```python
from build123d import *

# Parameters (mm, degrees)
SKETCH1_R           = 5
BOSS_EXTRUDE1_DEPTH = 40
CUT_EXTRUDE1_REACH  = 50.283
SKETCH3_W           = 23
SKETCH3_H           = 33
BOSS_EXTRUDE2_DEPTH = 3.5
CHAMFER1_SIZE       = 2
SKETCH6_R           = 5
CUT_EXTRUDE8_DEPTH  = 52.53882032


with BuildPart() as part:
    # Sketch1 → Boss-Extrude1 (new body)
    with BuildSketch(Plane.XY):
        with BuildLine():
            ThreePointArc((-5.590169944, -10), (0, -12.5), (5.590169944, -10))
            Line((5.590169944, -10), (15, -10))
            Line((15, -10), (15, 10))
            Line((15, 10), (-15, 10))
            Line((-15, 10), (-15, -10))
            Line((-15, -10), (-5.590169944, -10))
        make_face()
        with Locations((0, -5)):
            Circle(SKETCH1_R, mode=Mode.SUBTRACT)
    extrude(amount=BOSS_EXTRUDE1_DEPTH)

    # Sketch3 → Cut-Extrude1 (cut, up to next)
    with BuildSketch(Plane(origin=(0, 10, 0), x_dir=(1, 0, 0), z_dir=(0, 1, 0)), mode=Mode.PRIVATE) as cut_extrude1_sk1:
        with Locations((0, -20)):
            Rectangle(SKETCH3_W, SKETCH3_H)
    cut_extrude1_tool1 = extrude(cut_extrude1_sk1.sketch, amount=-CUT_EXTRUDE1_REACH, mode=Mode.PRIVATE) & part.part
    add(cut_extrude1_tool1.solids().sort_by_distance((0, 10, 20))[0], mode=Mode.SUBTRACT)

    # Sketch4 → Boss-Extrude2 (add)
    with BuildSketch(Plane.ZY.offset(15)):
        with BuildLine():
            Line((25.590169944, -10), (14.409830056, -10))
            ThreePointArc((14.409830056, -10), (20, -12.5), (25.590169944, -10))
        make_face()
    boss_extrude2 = extrude(amount=-BOSS_EXTRUDE2_DEPTH)

    # Mirror1: Boss-Extrude2 across plane
    add(boss_extrude2.mirror(Plane(origin=(0, 0, 0), x_dir=(0, 0, 1), z_dir=(1, 0, 0))))

    # Chamfer1
    chamfer1_edges = [part.edges().sort_by_distance(p)[0] for p in [
        (15, 0, 0),
        (-15, 10, 20),
        (15, 10, 20),
        (15, 0, 40),
        (0, 10, 40),
        (-15, 0, 40),
        (-11.5, 0, 36.5),
        (-11.5, 0, 3.5),
        (11.5, 0, 3.5),
        (11.5, 0, 36.5),
        (-15, 0, 0),
        (0, 10, 0),
    ]]
    chamfer(chamfer1_edges, length=CHAMFER1_SIZE)

    # Sketch6 → Cut-Extrude8 (cut, through all)
    with BuildSketch(Plane.ZY.offset(15)):
        with Locations(Location((20, -5, 0), (0, 0, 270))):
            Circle(SKETCH6_R)
    extrude(amount=-CUT_EXTRUDE8_DEPTH, mode=Mode.SUBTRACT)


solid = part.part
```
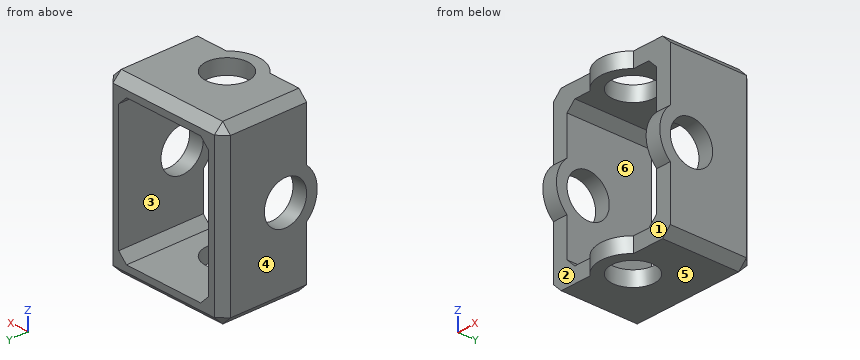
For this review, take the finished solid that the model builds, in its own axes (mm). Face numbers are marked on the shaded views. A direction names the side the tool comes from. Round coordinates to 2 decimals unless told otherwise and drop trailing zeros. Loops run counter-clockwise (first coordinate to the right, second up) from the corner with the lowest first, then second, coordinate; pieces in that order, holes last.
Q1. Add section D-D on z = 20. Write out the cut boundary in (x, y), plus the area to 3 significant figures.
Result sheet:
outline: (-15, -12.5) - (-11.5, -12.5) - (-11.5, -10) - (-15, -10) - close; (-15, 0) - (-11.5, 0) - (-11.5, 10) - (-13, 10) - (-15, 8) - close; (11.5, -12.5) - (15, -12.5) - (15, -10) - (11.5, -10) - close; (11.5, 0) - (15, 0) - (15, 8) - (13, 10) - (11.5, 10) - close
area: 83.5 mm2
Q2. Add section B-B on z = 36. Write out the cut boundary in (x, y).
Result sheet:
outline: (-15, -10) - (-10, -10) - (-10, 10) - (-13, 10) - (-15, 8) - close; (10, -10) - (15, -10) - (15, 8) - (13, 10) - (10, 10) - close
Q3. To check wall thickness, follow line 1 along X through (y, z) = (-2.25, 29.5); line 2 along Z through (x, y) = (-1.5, 4.25); line 3 along X through (y, z) = (-5, 2.5). State the ranges of each line that lie inside material, in increasing order.
Result sheet:
line 1: x = -15 to -11.5, 11.5 to 15
line 2: z = 0 to 3.5, 36.5 to 40
line 3: x = -15 to -5, 5 to 15
Q4. Machinability: for the marked faces 1, 2 and 3, which of the approach directions +Z, -Z, +X, -X, +Y, -Y give a long, thin tool a straight path to every point of the face, cutting with its end or side? Answer none if there is none.
Result sheet:
face 1: -Z, +X, -Y
face 2: -Z, -X, -Y
face 3: +Y, -Y
Q5. Insertion check: pin 1 Ø7.5 at (x, z) = (10, 36) entering from -Y. The pin has a flat end and moves straight along its axis. Give the tip position at first contact, or say it passes through.
Result sheet:
pin 1: stops at y = -10
Q6. Add section C-C on x = 0. Write out the cut boundary in (y, z), plus the area to 3 significant figures.
Result sheet:
outline: (-12.5, 0) - (-10, 0) - (-10, 3.5) - (-12.5, 3.5) - close; (-12.5, 36.5) - (-10, 36.5) - (-10, 40) - (-12.5, 40) - close; (0, 0) - (8, 0) - (10, 2) - (10, 3.5) - (0, 3.5) - close; (0, 36.5) - (10, 36.5) - (10, 38) - (8, 40) - (0, 40) - close
area: 83.5 mm2
Q7. Mouldability with a two-part tool opening along Z and no side actions: class the marked faces 4, 5 and 6 as +Z half, -Z half, draft (parallel to the pull), parting line (faces both ways), or undercut.
Result sheet:
face 4: draft
face 5: -Z half
face 6: undercut
Q8. Add section A-A on y = -1. Give the number of separate pieces and of enclosed holes in the cut face, plus the area to 3 significant figures.
Result sheet:
separate pieces: 4
enclosed holes: 0
area: 357 mm2
